Geometry: final body of the model. Coordinates: model frame, mm. A direction names the side the tool comes from. Coordinates: 2 decimals unless noted, no trailing zeros. Loops run counter-clockwise (first coordinate to the right, second up) from the corner with the lowest first, then second, coordinate; pieces in that order, holes last. Notation, with made-up numbers: (16.25, 49) - (29.25, 49) arc R22 ccw to (29.25, 59) - close; hole circle Ø4 at (-16.75, -37.5). An arc over 180 degrees is marked (long way). Return JSON: item names as keys, results as strings.
from build123d import *

# Parameters (mm, degrees)
F0_R     = 4.25
F1_DEPTH = 15
F2_R     = 1.65
F3_DEPTH = 20


with BuildPart() as f1:
    # F0 (on Top) → F1 (new body)
    with BuildSketch(Plane.XY):
        Polygon((-20, -60), (20, -60), (20, 0), (10, 20), (-10, 20), (-20, 0), align=None)
        Circle(F0_R, mode=Mode.SUBTRACT)
    extrude(amount=F1_DEPTH)

    # F2 (on face) → F3 (cut)
    with BuildSketch(Plane.XZ.offset(60)):
        with Locations((10, 7.5)):
            Circle(F2_R)
        with Locations((-10, 7.5)):
            Circle(F2_R)
    extrude(amount=-F3_DEPTH, mode=Mode.SUBTRACT)


solid = f1.part
Item 1: Section query D-D, the plane y = 12.5. Return loops of the section in (x, z), and give its area (4 significant figures).
Worked out:
{"outline": "(-13.75, 0) - (13.75, 0) - (13.75, 15) - (-13.75, 15) - close", "area": "412.5 mm^2"}
Item 2: Section query B-B, the plane y = -47. Return loops of the section in (x, z).
Worked out:
{"outline": "(-20, 0) - (20, 0) - (20, 15) - (-20, 15) - close; hole circle Ø3.3 at (-10, 7.5); hole circle Ø3.3 at (10, 7.5)"}
Item 3: Mould query, pull axis Z, two halves, no side actions, for faces 3 (the face through (10, -40, 8)), 4 (the face through (20, -30, 7)), 5 (the face through (0, -19, 15)), 6 (the face through (0, -19, 0)). Classes: +Z half, -Z half, draft (parallel to the pull), parting line (faces both ways), or undercut.
Worked out:
{"face 3": "undercut", "face 4": "draft", "face 5": "+Z half", "face 6": "-Z half"}
Item 4: Section query A-A, the plane z = 10.25. Return loops of the section in (x, y), and give its area (3 significant figures).
Worked out:
{"outline": "(-20, -60) - (20, -60) - (20, 0) - (10, 20) - (-10, 20) - (-20, 0) - close; hole circle Ø8.5 at (0, 0)", "area": "2,940 mm^2"}
Item 5: Section query C-C, the plane x = 3. Return loops of the section in (y, z), and give its area (3 significant figures).
Worked out:
{"outline": "(-60, 0) - (-3.01, 0) - (-3.01, 15) - (-60, 15) - close; (3.01, 0) - (20, 0) - (20, 15) - (3.01, 15) - close", "area": "1,110 mm^2"}
Item 6: Ray query, probe 1 along Z at (x, y) = (10, -46); probe 2 along Y at (x, z) = (0, 8); probe 3 along X at (y, z) = (1, 14). Return the intervals inside material, ascending. Write a range as from..to.
Worked out:
{"probe 1": "0..5.85, 9.15..15", "probe 2": "-60..-4.25, 4.25..20", "probe 3": "-19.5..-4.13, 4.13..19.5"}
Item 7: Reachability of faces 1 (the face through (-10, -40, 8)), 2 (the face through (0, 20, 7)) from +Z, -Z, +X, -X, +Y, -Y: full face, straight path, thin tool, end or side. Return the list, or none.
Worked out:
{"face 1": "-Y", "face 2": "+Z, -Z, +X, -X, +Y"}
Item 8: First-contact query: pin 1 Ø1 at (x, z) = (-9.5, 8) entering from -Y; pin 2 Ø5 at (x, z) = (14, 13) entering from +Y. Flat tips, straight axial feed; report the tip coordinate or a pass-through.
Worked out:
{"pin 1": "y = -40", "pin 2": "y = 17"}
